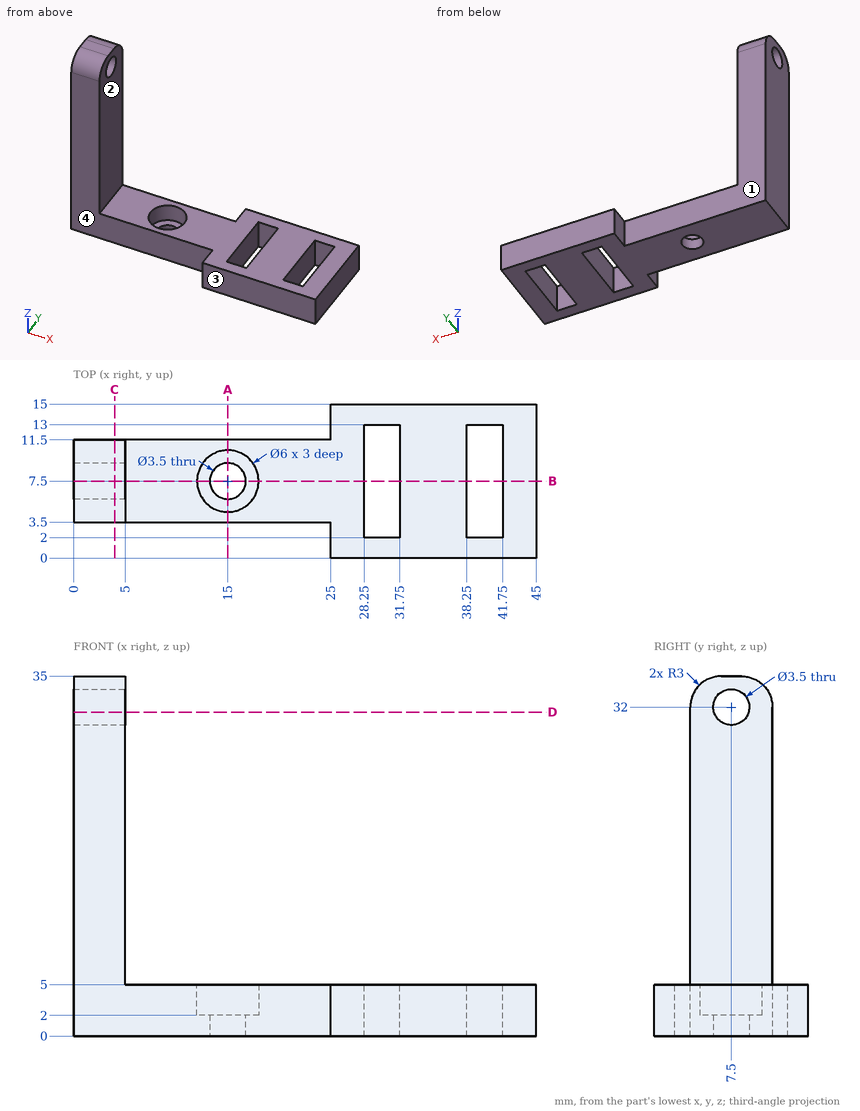
Here's the drawing with two shaded views (mm, measured from the low corner). I have some questions. A direction names the side the tool comes from. Coordinates: 2 decimals unless noted, no trailing zeros. Order: outer loops, then holes, each group sorted by start corner. A loop starts at its lowest first (then second) coordinate and runs counter-clockwise, first axis right, second up.
Q1. Please list where these lines run through material, in increasing order: L1, parallel to Y at x = 15, z = 0.4; L2, parallel to Y at x = 15, z = 3.3; L3, parallel to Z at x = 17.5, y = 9.
Q2. Suppose I cut it at C-C on x = 4. Please give me the cut outline in (y, z), and give its area (3 significant figures).
Q3. Which directions (+Z, -Z, +X, -X, +Y, -Y) give clear straight access to the entire face, cutting with the end or side of a thin tool? Please do the marked faces 1, 2, 3 and 4.
Q4. Will these pins go through, and if not, where does the flat tip stop? pin 1 (1.8 mm diameter, centred on y = 13.5, z = 2, fed in from -X); pin 2 (7.5 mm diameter, centred on x = 7.5, z = 8.5, fed in from +Y); pin 3 (8 mm diameter, centred on y = 12.5, z = 31.5, fed in from +X); pin 4 (1 mm diameter, centred on x = 24, y = 2.5, fed in from -Z).
Q5. Suppose I cut it at A-A on x = 15. Please give me the cut outline in (y, z).
Q6. Suppose I cut it at D-D on z = 31.5. Please give me the cut outline in (x, y), and give its area (3 significant figures).
Q7. Suppose I cut it at B-B on y = 7.5. Please give me the cut outline in (x, z).
Answer:
1. L1: y = 3.5 to 5.75, 9.25 to 11.5
1. L2: y = 3.5 to 4.5, 10.5 to 11.5
1. L3: z = 0 to 2
2. outline: (3.5, 0) - (11.5, 0) - (11.5, 32) arc R3 ccw to (8.5, 35) - (6.5, 35) arc R3 ccw to (3.5, 32) - close; hole circle Ø3.5 at (7.5, 32)
2. area: 267 mm2
3. face 1: +Z, -Z, -X, +Y
3. face 2: +Z, +X, +Y, -Y
3. face 3: +Z, -Z, +X, -X, -Y
3. face 4: +Z, -Z, -X, -Y
4. pin 1: stops at x = 25
4. pin 2: stops at y = 11.5
4. pin 3: stops at x = 5
4. pin 4: passes through
5. outline: (3.5, 0) - (5.75, 0) - (5.75, 2) - (4.5, 2) - (4.5, 5) - (3.5, 5) - close; (9.25, 0) - (11.5, 0) - (11.5, 5) - (10.5, 5) - (10.5, 2) - (9.25, 2) - close
6. outline: (0, 3.5) - (5, 3.5) - (5, 5.82) - (0, 5.82) - close; (0, 9.18) - (5, 9.18) - (5, 11.5) - (0, 11.5) - close
6. area: 23.2 mm2
7. outline: (0, 0) - (13.25, 0) - (13.25, 2) - (12, 2) - (12, 5) - (5, 5) - (5, 30.25) - (0, 30.25) - close; (0, 33.75) - (5, 33.75) - (5, 35) - (0, 35) - close; (16.75, 0) - (28.25, 0) - (28.25, 5) - (18, 5) - (18, 2) - (16.75, 2) - close; (31.75, 0) - (38.25, 0) - (38.25, 5) - (31.75, 5) - close; (41.75, 0) - (45, 0) - (45, 5) - (41.75, 5) - close
